```python
from build123d import *

# Parameters (mm, degrees)
F1_DEPTH       = 70
F3_D           = 3.5
F3_CBORE_D     = 6
F3_CBORE_DEPTH = 4.5


with BuildPart() as f1:
    # F0 (on Front) → F1 (new body)
    with BuildSketch(Plane.XZ):
        with BuildLine():
            Line((-1.510102, -5), (6.792893, -5))
            Line((6.792893, -5), (7.5, -4.292893))
            Line((7.5, -4.292893), (7.5, 0.585786))
            ThreePointArc((7.5, 0.585786), (6.978027, 0.902015), (6.625227, 1.4))
            Line((6.625227, 1.4), (5.7, 1.4))
            Line((5.7, 1.4), (5.7, 2.6))
            Line((5.7, 2.6), (6.625227, 2.6))
            ThreePointArc((6.625227, 2.6), (6.978027, 3.097985), (7.5, 3.414214))
            Line((7.5, 3.414214), (7.5, 4.505025))
            Line((7.5, 4.505025), (7.005025, 5))
            Line((7.005025, 5), (-7.005025, 5))
            Line((-7.005025, 5), (-7.5, 4.505025))
            Line((-7.5, 4.505025), (-7.5, 3.414214))
            ThreePointArc((-7.5, 3.414214), (-6.978027, 3.097985), (-6.625227, 2.6))
            Line((-6.625227, 2.6), (-5.7, 2.6))
            Line((-5.7, 2.6), (-5.7, 1.4))
            Line((-5.7, 1.4), (-6.625227, 1.4))
            ThreePointArc((-6.625227, 1.4), (-6.978027, 0.902015), (-7.5, 0.585786))
            Line((-7.5, 0.585786), (-7.5, -4.292893))
            Line((-7.5, -4.292893), (-6.792893, -5))
            Line((-6.792893, -5), (-2.489898, -5))
            ThreePointArc((-2.489898, -5), (-2, -4.7), (-1.510102, -5))
        make_face()
    extrude(amount=F1_DEPTH)

    # F3 (through all)
    with Locations(Plane.XY.offset(5)):
        with Locations((0, -95), (0, -215), (0, -295), (0, -55), (0, -335), (0, -15), (0, -175), (0, -255), (0, -135), (0, -855), (0, -455), (0, -895), (0, -815), (0, -655), (0, -775), (0, -935), (0, -615), (0, -735), (0, -535), (0, -695), (0, -375), (0, -575), (0, -495), (0, -415), (0, -1175), (0, -1375), (0, -1215), (0, -1615), (0, -1095), (0, -1135), (0, -1655), (0, -1255), (0, -1055), (0, -1295), (0, -975), (0, -1535), (0, -1415), (0, -1695), (0, -1335), (0, -1575), (0, -1495), (0, -1015), (0, -1455), (0, -1895), (0, -1775), (0, -1735), (0, -1975), (0, -1935), (0, -1815), (0, -1855)):
            CounterBoreHole(F3_D / 2, F3_CBORE_D / 2, F3_CBORE_DEPTH)


solid = f1.part
```
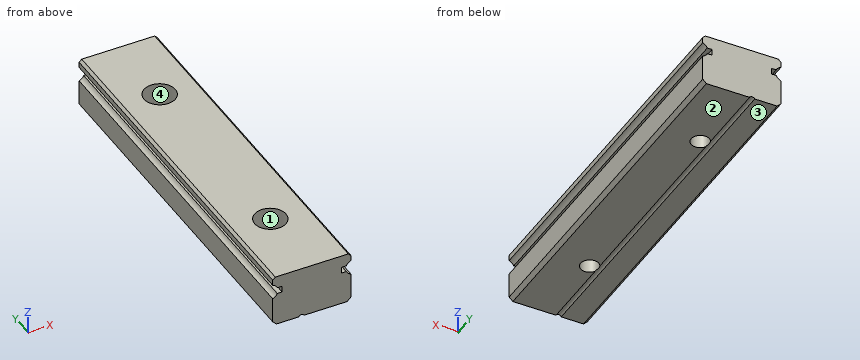
Could you check a few things on this model? Use its own coordinates, in mm. Face numbers are marked on the shaded views. A direction names the side the tool comes from. Coordinates: 2 decimals unless noted, no trailing zeros. Loops run counter-clockwise (first coordinate to the right, second up) from the corner with the lowest first, then second, coordinate; pieces in that order, holes last. Notation, with made-up numbers: M 71,-34.5 L 119,-34.5 A29 cw 119,-8.5 Z; hole C 55,40 d4. An arc over 180 degrees is marked long. Put each result on its own line as item: value. Start each with the question number.
(1) Suppose I cut it at D-D on y = -64. Please give me the cut outline in (x, z).
(2) Suppose I cut it at A-A on x = 0. Please give me the cut outline in (y, z), then the cut area to 4 significant figures.
(3) I need wall thicknesses on line 1 (Y direction, x = 0, z = 2.75); line 2 (Z direction, x = 6.25, y = -46); line 3 (Y direction, x = 0, z = -3.85). Which ranges of each line are inside material? Lowest first, please. Write a range as from..to.
(4) Will these pins go through, and if not, where does the flat tip stop? P1, Ø0.6, axis at y = -35, z = 2, coming from the +X side; P2, Ø3, axis at x = 0, y = -55, coming from the +Z side; P3, Ø0.6, axis at y = -52.5, z = 2, coming from the -X side.
(5) Suppose I cut it at B-B on z = -2.5. Please give me the cut outline in (x, y).
(6) Thinking about a two-plate mould opening in X: for the marked faces 1 and 2, which applies, pulls with the +X half, pulls with the -X half, needs draft (parallel to the pull), parting line crosses it, or undercut?
(7) For the marked faces 3 and 4, which set-ups out of +Z, -Z, +X, -X, +Y, -Y let a thin tool reach every point of the face, with its end or its side?
Solutions:
1. outline: M -7.5,-4.29 L -6.79,-5 L -2.49,-5 A0.55 cw -1.51,-5 L 6.79,-5 L 7.5,-4.29 L 7.5,0.59 A1.5 cw 6.63,1.4 L 5.7,1.4 L 5.7,2.6 L 6.63,2.6 A1.5 cw 7.5,3.41 L 7.5,4.51 L 7.01,5 L -7.01,5 L -7.5,4.51 L -7.5,3.41 A1.5 cw -6.63,2.6 L -5.7,2.6 L -5.7,1.4 L -6.63,1.4 A1.5 cw -7.5,0.59 Z
2. outline: M -70,-5 L -56.75,-5 L -56.75,0.5 L -58,0.5 L -58,5 L -70,5 Z; M -53.25,-5 L -16.75,-5 L -16.75,0.5 L -18,0.5 L -18,5 L -52,5 L -52,0.5 L -53.25,0.5 Z; M -13.25,-5 L 0,-5 L 0,5 L -12,5 L -12,0.5 L -13.25,0.5 Z
2. area: 607.5 mm2
3. line 1: y = -70..-58, -52..-18, -12..0
3. line 2: z = -5..1.4, 2.6..5
3. line 3: y = -70..-56.75, -53.25..-16.75, -13.25..0
4. P1: stops at x = 5.7
4. P2: passes through
4. P3: stops at x = -5.7
5. outline: M -7.5,-70 L 7.5,-70 L 7.5,0 L -7.5,0 Z; hole C 0,-55 d3.5; hole C 0,-15 d3.5
6. face 1: undercut
6. face 2: needs draft
7. face 3: -Z, +X, -X, +Y, -Y
7. face 4: +Z
